Solid Edge part; units mm, degrees
sketch "Sketch1" plane through (0, 0, 0) normal (0, 0, 1) x (1, 0, 0)
  line L0 (-5.9, -2.35) -> (5.9, -2.35)
  line L1 (5.9, -2.35) -> (5.9, 2.35)
  line L2 (5.9, 2.35) -> (-5.9, 2.35)
  line L3 (-5.9, 2.35) -> (-5.9, -2.35)
  circle A0 centre (0, 0) radius 1.15
extrude "Protrusion1" add sketch "Sketch1" along normal blind 5.9
properties material "Wood, Pine"
Check sheet for the modelled part. Datum: model origin and axes. Units: mm. Coordinates: 2 decimals unless noted, no trailing zeros. Write each loop counter-clockwise with the first axis right and the second up, starting at its lowest first coordinate (ties: lowest second). Pieces come first, ordered by that corner, then holes. Notation, with made-up numbers: M 27,66.5 L 45,66.5 A23 cw 45,91.5 Z; hole C -6.75,78.5 d9. An arc over 180 degrees is marked long. Write item = value, one per line. Start each with the question number.
1. Sectioned sample at A-A (x = 0). Record the cut outline in (y, z), then the cut area to 3 significant figures.
2. Sectioned sample at B-B (y = 0). Record the cut outline in (x, z).
3. Sectioned sample at C-C (z = 2.3). Record the cut outline in (x, y).
4. Thickness scan on probe 1 along Y at (x, z) = (0, 4.8); probe 2 along X at (y, z) = (-0.3, 5.3); probe 3 along Y at (x, z) = (-1, 4.25). Record the ranges inside material, lowest first.
5. Mould release check, pull along Y, two halves, no side actions. Record for faces 1 (the flat face through (0, 2.35, 3)), 2 (the cylindrical face through (-0.91, 0.7, 2.91)), 3 (the flat face through (-1.4, 0, 0)): pulls with the +Y half, pulls with the -Y half, needs draft (parallel to the pull), parting line crosses it, or undercut.
The answers:
q1.outline = M -2.35,0 L -1.15,0 L -1.15,5.9 L -2.35,5.9 Z; M 1.15,0 L 2.35,0 L 2.35,5.9 L 1.15,5.9 Z
q1.area = 14.2 mm²
q2.outline = M -5.9,0 L -1.15,0 L -1.15,5.9 L -5.9,5.9 Z; M 1.15,0 L 5.9,0 L 5.9,5.9 L 1.15,5.9 Z
q3.outline = M -5.9,-2.35 L 5.9,-2.35 L 5.9,2.35 L -5.9,2.35 Z; hole C 0,0 d2.3
q4.probe_1 = -2.35 to -1.15, 1.15 to 2.35
q4.probe_2 = -5.9 to -1.11, 1.11 to 5.9
q4.probe_3 = -2.35 to -0.57, 0.57 to 2.35
q5.face_1 = pulls with the +Y half
q5.face_2 = undercut
q5.face_3 = needs draft
